```python
from build123d import *

# Parameters (mm, degrees)
F0_R     = 1.1
F1_DEPTH = 1.5
F2_W     = 12
F2_H     = 24
F3_DEPTH = 1.5
F4_R     = 5
F5_DEPTH = 1.5


# Not quite as in the source:
# - a feature names something its author has since deleted; it is built from what else it names


with BuildPart() as f1:
    # F0 (on Top) → F1 (new body)
    with BuildSketch(Plane.XY):
        with BuildLine():
            Line((-5.7, -48), (6.3, -48))
            Line((6.3, -48), (6.3, -45))
            ThreePointArc((6.3, -45), (0.9721111048, -38.7754518236), (-6, -43.0790627288))
            ThreePointArc((-6, -43.0790627288), (-5.7754518236, -44.0278888952), (-5.7, -45))
            Line((-5.7, -45), (-5.7, -48))
        make_face()
        with Locations((-1.5, -45)):
            Circle(F0_R, mode=Mode.SUBTRACT)
        with BuildLine():
            Line((25.5, -48), (25.5, 48))
            Line((25.5, 48), (6.3, 48))
            Line((6.3, 48), (6.3, 45))
            ThreePointArc((6.3, 45), (0, 38.7), (-6.3, 45))
            Line((-6.3, 45), (-6.3, 48))
            Line((-6.3, 48), (-25.5, 48))
            Line((-25.5, 48), (-25.5, -48))
            Line((-25.5, -48), (-18.3, -48))
            Line((-18.3, -48), (-18.3, -45))
            ThreePointArc((-18.3, -45), (-12.9721111048, -38.7754518236), (-6, -43.0790627288))
            ThreePointArc((-6, -43.0790627288), (0.9721111048, -38.7754518236), (6.3, -45))
            Line((6.3, -45), (6.3, -48))
            Line((6.3, -48), (25.5, -48))
        make_face()
        with Locations((-22.5, -45)):
            Circle(F0_R, mode=Mode.SUBTRACT)
        with Locations((-22.5, -24)):
            Circle(F0_R, mode=Mode.SUBTRACT)
        with Locations((-10.5, -24)):
            Circle(F0_R, mode=Mode.SUBTRACT)
        with Locations((-1.5, -24)):
            Circle(F0_R, mode=Mode.SUBTRACT)
        with Locations((10.5, -45)):
            Circle(F0_R, mode=Mode.SUBTRACT)
        with Locations((10.5, -24)):
            Circle(F0_R, mode=Mode.SUBTRACT)
        with Locations((-10.5, 24)):
            Circle(F0_R, mode=Mode.SUBTRACT)
        with Locations((-10.5, 45)):
            Circle(F0_R, mode=Mode.SUBTRACT)
        with Locations((10.5, 24)):
            Circle(F0_R, mode=Mode.SUBTRACT)
        with Locations((10.5, 45)):
            Circle(F0_R, mode=Mode.SUBTRACT)
        with Locations((-10.5, -24)):
            Circle(F0_R)
        with Locations((10.5, -45)):
            Circle(F0_R)
        with Locations((10.5, -24)):
            Circle(F0_R)
    extrude(amount=F1_DEPTH)

    # F2 (on face) → F3 (cut, through all)
    with BuildSketch(Plane(origin=(0, 0, 0), x_dir=(1, 0, 0), z_dir=(0, 0, -1))):
        Polygon((-13.5, -24), (-25.5, 21), (-25.5, -24), align=None)
        Polygon((25.5, 48), (13.5, 48), (13.5, 24), (13.5, -21), (13.5, -48), (25.5, -48), align=None)
        with Locations((-19.5, -36)):
            Rectangle(F2_W, F2_H)
        with Locations((7.5, 36)):
            Rectangle(F2_W, F2_H)
        Polygon((13.5, 24), (1.5, 24), (13.5, -21), align=None)
    extrude(amount=-F3_DEPTH, mode=Mode.SUBTRACT)

    # F4 (on face) → F5 (cut, through all)
    with BuildSketch(Plane(origin=(0, 0, 0), x_dir=(1, 0, 0), z_dir=(0, 0, -1))):
        with Locations((-0.4, -21)):
            Circle(F4_R)
        with Locations((-11.6, 21)):
            Circle(F4_R)
        with Locations((-6, 0)):
            Circle(F4_R)
    extrude(amount=-F5_DEPTH, mode=Mode.SUBTRACT)


solid = f1.part
```
Check sheet for the modelled part. Datum: model origin and axes. Units: mm. Give positions to 0.01 mm unless a question says otherwise; leave off trailing zeros. Loops run counter-clockwise (first coordinate to the right, second up) from the corner with the lowest first, then second, coordinate; pieces in that order, holes last. Notation, with made-up numbers: M 24,86 L 77,86 A34 cw 77,124 Z; hole C -33.5,-32 d7. An arc over 180 degrees is marked long. Answer as CSV lines item,"result".
Item 1: Depth check by flat-ended pin: pin 1 Ø6 at (x, y) = (-17.5, 34.5) entering from +Z. Enter the tip coordinate at first touch or a pass-through.
Reply:
pin 1,"through"
Item 2: Sectioned sample at B-B, the plane z = 0.45. State how many separate pieces and enclosed holes the cut face has, then the cut area to 3 significant figures.
Reply:
separate pieces,"1"
enclosed holes,"11"
area,"2,160 mm^2"
Item 3: Sectioned sample at D-D, the plane x = 3. Enter the section's corners in (y, z) (3 decimals).
Reply:
outline,"M -18.375,0 L 17.334,0 L 17.334,1.5 L -18.375,1.5 Z; M 24.666,0 L 39.46,0 L 39.46,1.5 L 24.666,1.5 Z"
Item 4: Scan lines: L1, parallel to Y at x = 0, z = 1.4; L2, parallel to Y at x = -1.5, z = 0.95; L3, parallel to X at y = 21, z = 0.65. Record each from-to range of solid material in increasing order.
Reply:
L1,"-48 to 16.02, 25.98 to 38.7"
L2,"-48 to -46.1, -43.9 to -25.1, -22.9 to -2.18, 2.18 to 16.12, 25.88 to 38.88"
L3,"-14.3 to -5.4, 4.6 to 13.5"
Item 5: Draft check along X on faces 1 (the face through (-19.416, 1.815, 0.74)), 2 (the face through (-15, 1, 1.5)), 3 (the face through (-23.6, -45, 0.7)). Enter one of: pulls with the +X half, pulls with the -X half, needs draft (parallel to the pull), parting line crosses it, or undercut.
Reply:
face 1,"pulls with the -X half"
face 2,"needs draft"
face 3,"undercut"
Item 6: Sectioned sample at C-C, the plane y = 22. Enter the section's corners in (x, z).
Reply:
outline,"M -14.03,0 L -5.3,0 L -5.3,1.5 L -14.03,1.5 Z; M 4.5,0 L 13.5,0 L 13.5,1.5 L 4.5,1.5 Z"
Item 7: Sectioned sample at A-A, the plane x = -22.5. Enter the section's corners in (y, z).
Reply:
outline,"M -48,0 L -46.1,0 L -46.1,1.5 L -48,1.5 Z; M -43.9,0 L -25.1,0 L -25.1,1.5 L -43.9,1.5 Z; M -22.9,0 L -9.75,0 L -9.75,1.5 L -22.9,1.5 Z"
